Autodesk Fusion 360 part; units mm, degrees
sketch "スケッチ1" plane through (0, 0, 0) normal (0, 1, 0) x (1, 0, 0)
  line L0 (0, 0) -> (44, 0)
  line L1 (44, 0) -> (44, -15)
  line L2 (44, -15) -> (0, -15)
  line L3 (0, -15) -> (0, 0)
  dimension "d1" = 44
  dimension "d2" = 15
sketch "スケッチ2" plane through (0, 0, 0) normal (0, 0, 1) x (1, 0, 0)
  line L0 (0, 0) -> (44, 0)
  line L1 (44, 0) -> (44, 50)
  line L2 (44, 50) -> (0, 50)
  line L3 (0, 50) -> (0, 0)
  dimension "d3" = 44
  dimension "d4" = 50
extrude "押し出し1" add sketch "スケッチ1" along normal blind 5
extrude "押し出し2" add sketch "スケッチ2" against normal blind 5
fillet "フィレット1" radius 2 1 edges at (22, 0, -5)
sketch "スケッチ3" plane through (0, 0, 0) normal (0, 1, 0) x (1, 0, 0)
sketch "スケッチ4" plane through (0, 0, 0) normal (0, 1, 0) x (1, 0, 0)
  line L0 (6.3, -2.5) -> (6.3, -2.5)
  line L1 (9.3, -5.5) -> (9.3, -9.5)
  line L2 (6.3, -12.5) -> (6.3, -12.5)
  line L3 (3.3, -9.5) -> (3.3, -5.5)
  arc A0 (6.3, -2.5) -> (3.3, -5.5) centre (6.3, -5.5) ccw
  arc A1 (9.3, -5.5) -> (6.3, -2.5) centre (6.3, -5.5) ccw
  arc A2 (6.3, -12.5) -> (9.3, -9.5) centre (6.3, -9.5) ccw
  arc A3 (3.3, -9.5) -> (6.3, -12.5) centre (6.3, -9.5) ccw
  arc A4 (34.7, -9.5) -> (37.7, -12.5) centre (37.7, -9.5) ccw
  line L4 (37.7, -2.5) -> (37.7, -2.5)
  line L5 (34.7, -9.5) -> (34.7, -5.5)
  arc A5 (40.7, -5.5) -> (37.7, -2.5) centre (37.7, -5.5) ccw
  line L6 (40.7, -5.5) -> (40.7, -9.5)
  arc A6 (37.7, -12.5) -> (40.7, -9.5) centre (37.7, -9.5) ccw
  line L7 (37.7, -12.5) -> (37.7, -12.5)
  arc A7 (37.7, -2.5) -> (34.7, -5.5) centre (37.7, -5.5) ccw
  point P0 (3.3, -2.5)
  point P1 (9.3, -2.5)
  point P2 (3.3, -12.5)
  point P3 (34.7, -2.5)
  point P4 (40.7, -2.5)
  point P5 (34.7, -12.5)
  dimension "d11" = 6
  dimension "d12" = 10
  dimension "d13" = 3
  dimension "d14" = 6
  dimension "d15" = 10
  dimension "d16" = 3
extrude "押し出し3" cut sketch "スケッチ4" along normal blind 5
sketch "スケッチ5" plane through (0, 0, 0) normal (0, 0, 1) x (1, 0, 0)
  circle A0 centre (9.25, 16) radius 2.75
  circle A1 centre (34.75, 16) radius 2.75
  circle A2 centre (21.45, 41.581) radius 2.75
  dimension "d19" = 5.5
  dimension "d20" = 5.5
  dimension "d21" = 5.5
extrude "押し出し5" cut sketch "スケッチ5" against normal blind 5
extrude "押し出し4" [suppressed]
Source: CAD feature listing. Evaluate the final solid. Frame: model axes, mm. A direction names the side the tool comes from. Coordinates: 2 decimals unless noted, no trailing zeros. Write each loop counter-clockwise with the first axis right and the second up, starting at its lowest first coordinate (ties: lowest second). Pieces come first, ordered by that corner, then holes. Notation, with made-up numbers: M 35,12.5 L 68,12.5 A11 ccw 68,25.5 Z; hole C -22.5,-36 d6. An arc over 180 degrees is marked long. Answer as a JSON object with one key per item and string values.
1. Contact query for flat-ended pins moving along their axis: P1, Ø5, axis at x = 20, y = 41, coming from the +Z side; P2, Ø7.5, axis at x = 13.5, z = 4, coming from the +Y side; P3, Ø8, axis at y = 23.5, z = 5, coming from the -X side. Output: stop coordinate, or through.
Evaluation:
{"P1": "z = 0", "P2": "y = 5", "P3": "through"}
2. Draft query along Y for faces 1 (the cylindrical face through (32, 16, -2)), 2 (the flat face through (3.3, 2, 8)), 3 (the flat face through (22, 5, 7)). Return one class per face: released by +Y, released by -Y, zero draft, split by the parting line, or undercut.
Evaluation:
{"face 1": "undercut", "face 2": "zero draft", "face 3": "released by +Y"}
3. Cut plane D-D on x = 14.5. Output: boundary loops of the cut face in (y, z), plus the area to 3 significant figures.
Evaluation:
{"outline": "M 0,-3 A2 ccw 2,-5 L 50,-5 L 50,0 L 5,0 L 5,15 L 0,15 Z", "area": "324 mm^2"}
4. Cut plane C-C on y = 16. Output: boundary loops of the cut face in (x, z).
Evaluation:
{"outline": "M 0,-5 L 6.5,-5 L 6.5,0 L 0,0 Z; M 12,-5 L 32,-5 L 32,0 L 12,0 Z; M 37.5,-5 L 44,-5 L 44,0 L 37.5,0 Z"}
5. Ray query, L1, parallel to X at y = 13.5, z = -2.75; L2, parallel to Y at x = 9.25, z = -1.05; L3, parallel to Z at x = 13.5, y = 37. Return the intervals inside material, ascending.
Evaluation:
{"L1": "0 to 8.1, 10.4 to 33.6, 35.9 to 44", "L2": "0 to 13.25, 18.75 to 50", "L3": "-5 to 0"}
6. Access query for faces 4 (the flat face through (22, 2, 15)), 5 (the flat face through (34.7, 2, 8)), 6 (the flat face through (22, 28, 0)). Directions: +Z, -Z, +X, -X, +Y, -Y. A direction counts if a zero-diameter tool reaches every point of the face in a straight line with its end or side. Return the directions, or none.
Evaluation:
{"face 4": "+Z, +X, -X, +Y, -Y", "face 5": "+Y, -Y", "face 6": "+Z, +X, -X, +Y"}
7. Cut plane A-A on z = 7.25. Output: boundary loops of the cut face in (x, y), plus the area to 3 significant figures.
Evaluation:
{"outline": "M 0,0 L 3.3,0 L 3.3,5 L 0,5 Z; M 9.3,0 L 34.7,0 L 34.7,5 L 9.3,5 Z; M 40.7,0 L 44,0 L 44,5 L 40.7,5 Z", "area": "160 mm^2"}
8. Cut plane B-B on x = 21.45. Output: boundary loops of the cut face in (y, z), plus the area to 3 significant figures.
Evaluation:
{"outline": "M 0,-3 A2 ccw 2,-5 L 38.83,-5 L 38.83,0 L 5,0 L 5,15 L 0,15 Z; M 44.33,-5 L 50,-5 L 50,0 L 44.33,0 Z", "area": "297 mm^2"}
